Drawing for the job (mm, zero at the part's lowest x, y, z). A direction names the side the tool comes from. Give positions to 0.01 mm unless a question says otherwise; leave off trailing zeros. Loops run counter-clockwise (first coordinate to the right, second up) from the corner with the lowest first, then second, coordinate; pieces in that order, holes last. Notation, with made-up numbers: M 70.5,-20 L 113.5,-20 A37 ccw 113.5,18 Z; hole C 83,33.25 d9. An arc over 180 degrees is marked long. Use CSV: the item, a comma, the result in double quotes. Start each with the question number.
(1) Slice it at A-A on x = 76.5. List the corners of the cut face in (y, z), and give its area (3 significant figures).
(2) Slice it at D-D on x = 114. List the corners of the cut face in (y, z).
(3) Tool access for the marked faces 1, 2, 3, 4 and 5: list every direction of +Z, -Z, +X, -X, +Y, -Y with a clear straight run to the whole face (end or side of a thin tool).
(4) Two-plate mould, pull along X, no slides. Class the marked faces 6, 7, 8 and 9: pulls with the +X half, pulls with the -X half, needs draft (parallel to the pull), parting line crosses it, or undercut.
(5) Wall check: line 1 along Z through (x, y) = (104.5, 63.5); line 2 along Y through (x, z) = (89, 136); line 3 along Y through (x, z) = (70, 55). Give the ranges that are in metal, low to high. Write a range as from..to.
(6) Slice it at C-C on z = 127. List the corners of the cut face in (x, y), and give its area (3 significant figures).
(7) Flat gauge pins, fed straight in: P1, Ø15, axis at x = 111, y = 77.07, coming from the +Z side (3 decimals); P2, Ø2, axis at x = 31.5, z = 20, coming from the -Y side; P3, Ø4, axis at x = 109, z = 48, coming from the +Y side (1 decimal); P4, Ø5, axis at x = 24.5, y = 105, coming from the +Z side. Where does each tip first touch, or does it go through?
(8) Slice it at B-B on y = 47.5. List the corners of the cut face in (x, z) (1 decimal).
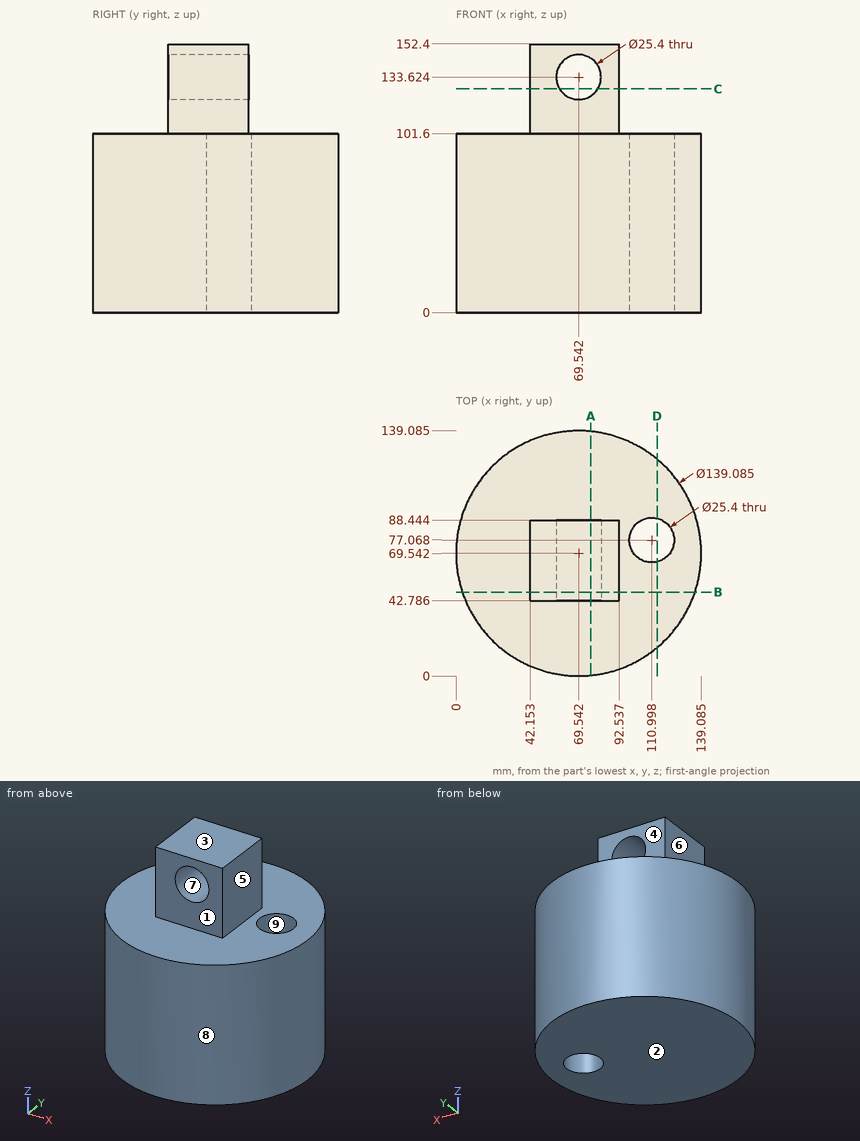
Reply:
1,outline,"M 0.35,0 L 138.74,0 L 138.74,101.6 L 88.44,101.6 L 88.44,123 L 42.79,123 L 42.79,101.6 L 0.35,101.6 Z; M 42.79,144.25 L 88.44,144.25 L 88.44,152.4 L 42.79,152.4 Z"
1,area,"15,400 mm^2"
2,outline,"M 16.07,0 L 64.73,0 L 64.73,101.6 L 16.07,101.6 Z; M 89.41,0 L 123.02,0 L 123.02,101.6 L 89.41,101.6 Z"
3,face 1,"+Z, +X, -X, -Y"
3,face 2,"-Z, +X, -X, +Y, -Y"
3,face 3,"+Z, +X, -X, +Y, -Y"
3,face 4,"+Z, +X, -X, +Y"
3,face 5,"+Z, +X, +Y, -Y"
4,face 6,"pulls with the -X half"
4,face 7,"undercut"
4,face 8,"parting line crosses it"
4,face 9,"undercut"
5,line 1,"z = 0..101.6"
5,line 2,"y = 42.79..88.44"
5,line 3,"y = 0..139.08"
6,outline,"M 42.15,42.79 L 58.71,42.79 L 58.71,88.44 L 42.15,88.44 Z; M 80.38,42.79 L 92.54,42.79 L 92.54,88.44 L 80.38,88.44 Z"
6,area,"1,310 mm^2"
7,P1,"passes through"
7,P2,"stops at y = 10.69"
7,P3,"stops at y = 128.1"
7,P4,"stops at z = 101.6"
8,outline,"M 3.6,0 L 135.5,0 L 135.5,101.6 L 92.5,101.6 L 92.5,152.4 L 42.2,152.4 L 42.2,101.6 L 3.6,101.6 Z; hole C 69.5,133.6 d25.4"
